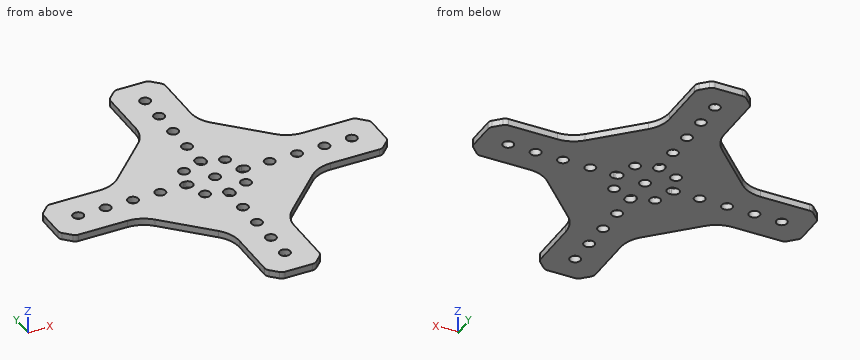
from build123d import *

# Parameters (mm, degrees)
SKETCH1_R           = 2.4892
BOSS_EXTRUDE1_DEPTH = 3.175


with BuildPart() as part:
    # Sketch1 → Boss-Extrude1 (new body)
    with BuildSketch(Plane(origin=(0, 0, 0), x_dir=(-1, 0, 0), z_dir=(0, 0, -1))):
        with BuildLine():
            Line((-59.897474683, 25.4), (-82.657359313, 25.4))
            ThreePointArc((-82.657359313, 25.4), (-83.80540961, 25.171638598), (-84.778679656, 24.521320344))
            Line((-84.778679656, 24.521320344), (-88.021320344, 21.278679656))
            ThreePointArc((-88.021320344, 21.278679656), (-88.671638598, 20.30540961), (-88.9, 19.157359313))
            Line((-88.9, 19.157359313), (-88.9, 6.242640687))
            ThreePointArc((-88.9, 6.242640687), (-88.671638598, 5.09459039), (-88.021320344, 4.121320344))
            Line((-88.021320344, 4.121320344), (-84.778679656, 0.878679656))
            ThreePointArc((-84.778679656, 0.878679656), (-83.80540961, 0.228361402), (-82.657359313, 0))
            Line((-82.657359313, 0), (-59.897474683, 0))
            ThreePointArc((-59.897474683, 0), (-54.157223198, -1.141807012), (-49.290872965, -4.393398282))
            Line((-49.290872965, -4.393398282), (-29.793398282, -23.890872965))
            ThreePointArc((-29.793398282, -23.890872965), (-26.541807012, -28.757223198), (-25.4, -34.497474683))
            Line((-25.4, -34.497474683), (-25.4, -57.257359313))
            ThreePointArc((-25.4, -57.257359313), (-25.171638598, -58.40540961), (-24.521320344, -59.378679656))
            Line((-24.521320344, -59.378679656), (-21.278679656, -62.621320344))
            ThreePointArc((-21.278679656, -62.621320344), (-20.30540961, -63.271638598), (-19.157359313, -63.5))
            Line((-19.157359313, -63.5), (-6.242640687, -63.5))
            ThreePointArc((-6.242640687, -63.5), (-5.09459039, -63.271638598), (-4.121320344, -62.621320344))
            Line((-4.121320344, -62.621320344), (-0.878679656, -59.378679656))
            ThreePointArc((-0.878679656, -59.378679656), (-0.228361402, -58.40540961), (0, -57.257359313))
            Line((0, -57.257359313), (0, -34.497474683))
            ThreePointArc((0, -34.497474683), (1.141807012, -28.757223198), (4.393398282, -23.890872965))
            Line((4.393398282, -23.890872965), (23.890872965, -4.393398282))
            ThreePointArc((23.890872965, -4.393398282), (28.757223198, -1.141807012), (34.497474683, 0))
            Line((34.497474683, 0), (57.257359313, 0))
            ThreePointArc((57.257359313, 0), (58.40540961, 0.228361402), (59.378679656, 0.878679656))
            Line((59.378679656, 0.878679656), (62.621320344, 4.121320344))
            ThreePointArc((62.621320344, 4.121320344), (63.271638598, 5.09459039), (63.5, 6.242640687))
            Line((63.5, 6.242640687), (63.5, 19.157359313))
            ThreePointArc((63.5, 19.157359313), (63.271638598, 20.30540961), (62.621320344, 21.278679656))
            Line((62.621320344, 21.278679656), (59.378679656, 24.521320344))
            ThreePointArc((59.378679656, 24.521320344), (58.40540961, 25.171638598), (57.257359313, 25.4))
            Line((57.257359313, 25.4), (34.497474683, 25.4))
            ThreePointArc((34.497474683, 25.4), (28.757223198, 26.541807012), (23.890872965, 29.793398282))
            Line((23.890872965, 29.793398282), (4.393398282, 49.290872965))
            ThreePointArc((4.393398282, 49.290872965), (1.141807012, 54.157223198), (0, 59.897474683))
            Line((0, 59.897474683), (0, 82.657359313))
            ThreePointArc((0, 82.657359313), (-0.228361402, 83.80540961), (-0.878679656, 84.778679656))
            Line((-0.878679656, 84.778679656), (-4.121320344, 88.021320344))
            ThreePointArc((-4.121320344, 88.021320344), (-5.09459039, 88.671638598), (-6.242640687, 88.9))
            Line((-6.242640687, 88.9), (-19.157359313, 88.9))
            ThreePointArc((-19.157359313, 88.9), (-20.30540961, 88.671638598), (-21.278679656, 88.021320344))
            Line((-21.278679656, 88.021320344), (-24.521320344, 84.778679656))
            ThreePointArc((-24.521320344, 84.778679656), (-25.171638598, 83.80540961), (-25.4, 82.657359313))
            Line((-25.4, 82.657359313), (-25.4, 59.897474683))
            ThreePointArc((-25.4, 59.897474683), (-26.541807012, 54.157223198), (-29.793398282, 49.290872965))
            Line((-29.793398282, 49.290872965), (-49.290872965, 29.793398282))
            ThreePointArc((-49.290872965, 29.793398282), (-54.157223198, 26.541807012), (-59.897474683, 25.4))
        make_face()
        with Locations((-12.7, -12.7)):
            Circle(SKETCH1_R, mode=Mode.SUBTRACT)
        with Locations((-12.7, -38.1)):
            Circle(SKETCH1_R, mode=Mode.SUBTRACT)
        with Locations((-12.7, -25.4)):
            Circle(SKETCH1_R, mode=Mode.SUBTRACT)
        with Locations((-12.7, -50.8)):
            Circle(SKETCH1_R, mode=Mode.SUBTRACT)
        with Locations((-12.7, 12.7)):
            Circle(SKETCH1_R, mode=Mode.SUBTRACT)
        with Locations((-63.5, 12.7)):
            Circle(SKETCH1_R, mode=Mode.SUBTRACT)
        with Locations((-38.1, 12.7)):
            Circle(SKETCH1_R, mode=Mode.SUBTRACT)
        with Locations((-76.2, 12.7)):
            Circle(SKETCH1_R, mode=Mode.SUBTRACT)
        with Locations((-50.8, 12.7)):
            Circle(SKETCH1_R, mode=Mode.SUBTRACT)
        with Locations((25.4, 12.7)):
            Circle(SKETCH1_R, mode=Mode.SUBTRACT)
        with Locations((50.8, 12.7)):
            Circle(SKETCH1_R, mode=Mode.SUBTRACT)
        with Locations((12.7, 12.7)):
            Circle(SKETCH1_R, mode=Mode.SUBTRACT)
        with Locations((38.1, 12.7)):
            Circle(SKETCH1_R, mode=Mode.SUBTRACT)
        with Locations((-12.7, 50.8)):
            Circle(SKETCH1_R, mode=Mode.SUBTRACT)
        with Locations((-12.7, 63.5)):
            Circle(SKETCH1_R, mode=Mode.SUBTRACT)
        with Locations((-12.7, 38.1)):
            Circle(SKETCH1_R, mode=Mode.SUBTRACT)
        with Locations((-12.7, 76.2)):
            Circle(SKETCH1_R, mode=Mode.SUBTRACT)
        with Locations((-3.175, 3.175)):
            Circle(SKETCH1_R, mode=Mode.SUBTRACT)
        with Locations((-22.225, 3.175)):
            Circle(SKETCH1_R, mode=Mode.SUBTRACT)
        with Locations((-22.225, 22.225)):
            Circle(SKETCH1_R, mode=Mode.SUBTRACT)
        with Locations((-3.175, 22.225)):
            Circle(SKETCH1_R, mode=Mode.SUBTRACT)
        with BuildLine():
            Line((0, 15.1892), (0.770384182, 15.1892))
            ThreePointArc((0.770384182, 15.1892), (3.259584182, 12.7), (0.770384182, 10.2108))
            Line((0.770384182, 10.2108), (0, 10.2108))
            ThreePointArc((0, 10.2108), (-2.4892, 12.7), (0, 15.1892))
        make_face(mode=Mode.SUBTRACT)
        with BuildLine():
            Line((-26.170384182, 15.1892), (-25.4, 15.1892))
            ThreePointArc((-25.4, 15.1892), (-22.9108, 12.7), (-25.4, 10.2108))
            Line((-25.4, 10.2108), (-26.170384182, 10.2108))
            ThreePointArc((-26.170384182, 10.2108), (-28.659584182, 12.7), (-26.170384182, 15.1892))
        make_face(mode=Mode.SUBTRACT)
        with BuildLine():
            Line((-15.1892, -0.770384182), (-15.1892, 0))
            ThreePointArc((-15.1892, 0), (-12.7, 2.4892), (-10.2108, 0))
            Line((-10.2108, 0), (-10.2108, -0.770384182))
            ThreePointArc((-10.2108, -0.770384182), (-12.7, -3.259584182), (-15.1892, -0.770384182))
        make_face(mode=Mode.SUBTRACT)
        with BuildLine():
            Line((-10.2108, 26.170384182), (-10.2108, 25.4))
            ThreePointArc((-10.2108, 25.4), (-12.7, 22.9108), (-15.1892, 25.4))
            Line((-15.1892, 25.4), (-15.1892, 26.170384182))
            ThreePointArc((-15.1892, 26.170384182), (-12.7, 28.659584182), (-10.2108, 26.170384182))
        make_face(mode=Mode.SUBTRACT)
    extrude(amount=-BOSS_EXTRUDE1_DEPTH)


solid = part.part
Input: part model. Units: mm. Frame: model coordinates. Give positions to 0.01 mm unless a question says otherwise; leave off trailing zeros. Order: outer loops, then holes, each group sorted by start corner. A loop starts at its lowest first (then second) coordinate and runs counter-clockwise, first axis right, second up.
Q1. Contact query for flat-ended pins moving along their axis: pin 1 Ø1.6 at (x, z) = (-51.5, 1) entering from +Y; pin 2 Ø1.5 at (y, z) = (36.5, 0.5) entering from -X; pin 3 Ø1.6 at (y, z) = (-46.5, 1.5) entering from +X. Output: stop coordinate, or through.
Checked values:
pin 1: stops at y = 25.4
pin 2: stops at x = -17.93
pin 3: stops at x = 25.4
Q2. Ray query, probe 1 along Y at (x, z) = (-38.1, 2.2); probe 2 along X at (y, z) = (-34, 1.55); probe 3 along X at (y, z) = (-49, 0.3). Return the intervals inside material, ascending.
Checked values:
probe 1: y = 0 to 10.21, 15.19 to 25.4
probe 2: x = -0.01 to 25.41
probe 3: x = 0 to 10.98, 14.42 to 25.4
Q3. Section B-B on x = -12.7. Output: boundary loops of the cut face in (y, z) (3 decimals).
Checked values:
outline: (-15.584, 0) - (10.211, 0) - (10.211, 3.175) - (-15.584, 3.175) - close; (15.189, 0) - (40.984, 0) - (40.984, 3.175) - (15.189, 3.175) - close
Q4. Section D-D on x = -45. Output: boundary loops of the cut face in (y, z) (3 decimals).
Checked values:
outline: (0, 0) - (25.4, 0) - (25.4, 3.175) - (0, 3.175) - close
Q5. Section C-C on z = 1.15. State how many separate pieces and enclosed holes the cut face has, and give its area (3 significant figures).
Checked values:
separate pieces: 1
enclosed holes: 25
area: 8,130 mm2
Q6. Section A-A on x = 76.2. Output: boundary loops of the cut face in (y, z) (3 decimals), and give its area (3 significant figures).
Checked values:
outline: (0, 0) - (10.211, 0) - (10.211, 3.175) - (0, 3.175) - close; (15.189, 0) - (25.4, 0) - (25.4, 3.175) - (15.189, 3.175) - close
area: 64.8 mm2
